Here's how the part is built. I have some questions about the finished solid (model axes, mm). A direction names the side the tool comes from. Give positions to 0.01 mm unless a question says otherwise; leave off trailing zeros. Write each loop counter-clockwise with the first axis right and the second up, starting at its lowest first coordinate (ties: lowest second). Pieces come first, ordered by that corner, then holes. Notation, with made-up numbers: (-34.5, -5) -> (12.5, -5) arc R24 cw to (12.5, 12) -> close; hole circle Ø4 at (-25, 83). An arc over 180 degrees is marked (long way). Return JSON: item names as keys, results as strings.
from build123d import *

# Parameters (mm, degrees)
FILLET1_R          = 1.5875
SKETCH2_R          = 4.7625
CUT_EXTRUDE2_DEPTH = 68.160068865
CHAMFER1_SIZE      = 1.27


with BuildPart() as part:
    # Sketch1 → Revolve1 (revolve)
    with BuildSketch(Plane.XY, mode=Mode.PRIVATE) as revolve1_sk:
        Polygon((0, 0), (0, 9.525), (25.4, 9.525), (25.4, 4.7625), (63.5, 4.7625), (63.5, 0), align=None)
    revolve(revolve1_sk.sketch.rotate(Axis((-10.444266115, 0, 0), (1, 0, 0)), 90), axis=Axis((-10.444266115, 0, 0), (1, 0, 0)))

    # Fillet1
    fillet1_edges = [part.edges().sort_by_distance(p)[0] for p in [
        (25.4, 0, -9.525),
        (0, 0, -9.525),
    ]]
    fillet(fillet1_edges, radius=FILLET1_R)

    # Sketch2 → Cut-Extrude2 (cut, through all)
    with BuildSketch(Plane.XY.offset(10.16)):
        with Locations((9.525, 0)):
            Circle(SKETCH2_R)
    extrude(amount=-CUT_EXTRUDE2_DEPTH, mode=Mode.SUBTRACT)

    # Chamfer1
    chamfer1_edges = [part.edges().sort_by_distance(p)[0] for p in [
        (63.5, 0, -4.7625),
    ]]
    chamfer(chamfer1_edges, length=CHAMFER1_SIZE)


solid = part.part
1. For pin 1 Ø1 at (x, y) = (20, 3) entering from +Z; pin 2 Ø3 at (x, z) = (26.5, 2.5) entering from +Y; pin 3 Ø10 at (x, y) = (52, 6) entering from +Z, each with a flat end and sliding along its axis, tell me the tip position at first contact or that it passes through.
Taken from the geometry:
{"pin 1": "stops at z = 9.19", "pin 2": "stops at y = 8.68", "pin 3": "stops at z = 4.66"}
2. If I drill on line 1 (X direction, y = 0, z = 2.5); line 2 (X direction, y = 0, z = -5.25); line 3 (Z direction, x = 51.5, y = -3.25), over which ranges is the centre line in solid material (lowest first)? Write a range as [from, to].
Taken from the geometry:
{"line 1": "x = [0, 4.76], [14.29, 63.5]", "line 2": "x = [0, 4.76], [14.29, 25.4]", "line 3": "z = [-3.48, 3.48]"}
3. If we mould it in two halves opening along Y, with no side actions, what happens to faces 3 (the face through (12.085, 4.016, 0.133)), 4 (the face through (44.07, 4.65, -1.03)), 5 (the face through (0, 0, 0))? For each: released by +Y, released by -Y, zero draft, split by the parting line, or undercut.
Taken from the geometry:
{"face 3": "undercut", "face 4": "split by the parting line", "face 5": "zero draft"}
4. Suppose I cut it at A-A, the plane y = 0. List the corners of the cut face in (x, z) for me (1 decimal).
Taken from the geometry:
{"outline": "(0, -7.9) arc R1.6 ccw to (1.6, -9.5) -> (4.8, -9.5) -> (4.8, 9.5) -> (1.6, 9.5) arc R1.6 ccw to (0, 7.9) -> close; (14.3, -9.5) -> (23.8, -9.5) arc R1.6 ccw to (25.4, -7.9) -> (25.4, -4.8) -> (62.2, -4.8) -> (63.5, -3.5) -> (63.5, 3.5) -> (62.2, 4.8) -> (25.4, 4.8) -> (25.4, 7.9) arc R1.6 ccw to (23.8, 9.5) -> (14.3, 9.5) -> close"}
5. Suppose I cut it at C-C, the plane x = 54.5. List the corners of the cut face in (y, z) for me (1 decimal).
Taken from the geometry:
{"outline": "circle Ø9.5 at (0, 0)"}
6. Which directions (+Z, -Z, +X, -X, +Y, -Y) give clear straight access to the entire face, cutting with the end or side of a thin tool? Please do faces 1 (the face through (12.856, 5.796, -7.559)), 2 (the face through (25.4, 5, 0)).
Taken from the geometry:
{"face 1": "+X, -X", "face 2": "+X"}
7. Suppose I cut it at B-B, the plane z = 0. List the corners of the cut face in (x, y) for me (1 decimal).
Taken from the geometry:
{"outline": "(0, -7.9) arc R1.6 ccw to (1.6, -9.5) -> (23.8, -9.5) arc R1.6 ccw to (25.4, -7.9) -> (25.4, -4.8) -> (62.2, -4.8) -> (63.5, -3.5) -> (63.5, 3.5) -> (62.2, 4.8) -> (25.4, 4.8) -> (25.4, 7.9) arc R1.6 ccw to (23.8, 9.5) -> (1.6, 9.5) arc R1.6 ccw to (0, 7.9) -> close; hole circle Ø9.5 at (9.5, 0)"}
